Could you check a few things on this drawing? It's one solid part, dimensions in mm from its lowest x, y, z. Round coordinates to 2 decimals unless told otherwise and drop trailing zeros. Write each loop counter-clockwise with the first axis right and the second up, starting at its lowest first coordinate (ties: lowest second). Pieces come first, ordered by that corner, then holes. Notation, with made-up numbers: (-13, 55.25) - (8, 55.25) arc R33 cw to (8, 87.25) - close; hole circle Ø7 at (80, 81). An arc over 180 degrees is marked (long way). One line per question, with ' | ' between items. Start each with the question number.
(1) If I drill on L1, parallel to Y at x = 9, z = 1.55; L2, parallel to X at y = 63.5, z = 3.95, over which ranges is the centre line in solid material (lowest first)?
(2) Imagine slicing it at A-A (y = 9). Write out the boundary of the cut face in (x, z).
(3) Will this pin go through, and if not, where does the flat tip stop? pin 1 (5 mm diameter, centred on x = 9, y = 9, fed in from -Z).
(4) Imagine slicing it at C-C (z = 4.05). Write out the boundary of the cut face in (x, y).
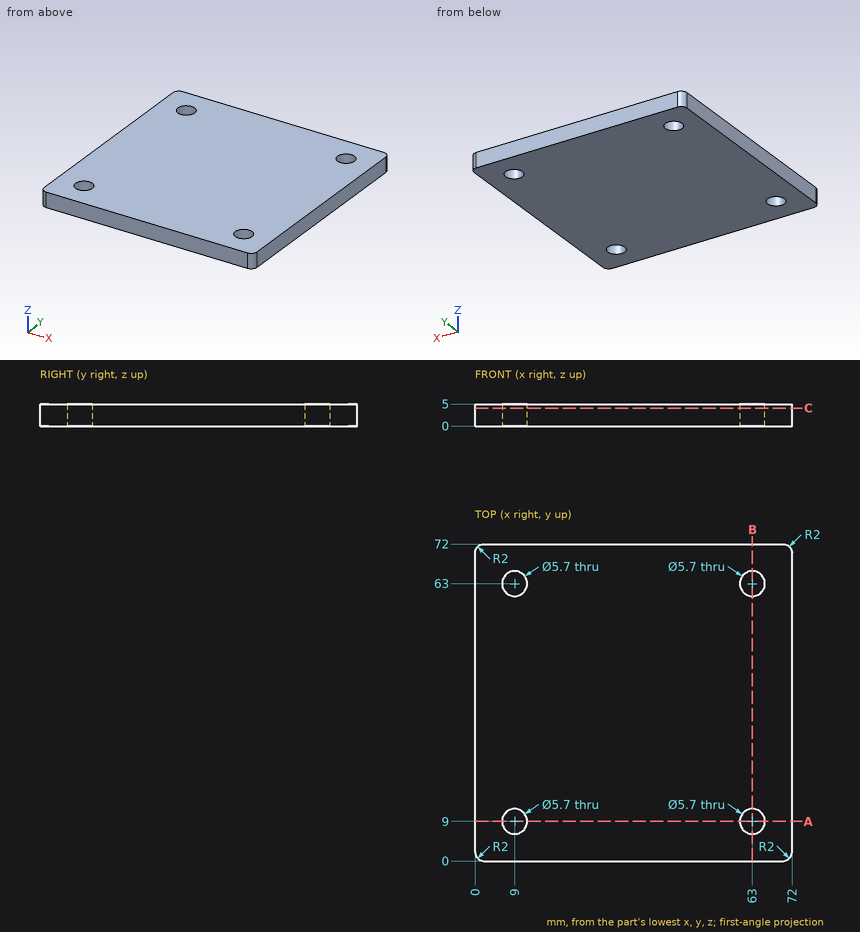
Check sheet entries:
1) L1: 0 to 6.15, 11.85 to 60.15, 65.85 to 72 | L2: 0 to 6.19, 11.81 to 60.19, 65.81 to 72
2) outline: (0, 0) - (6.15, 0) - (6.15, 5) - (0, 5) - close; (11.85, 0) - (60.15, 0) - (60.15, 5) - (11.85, 5) - close; (65.85, 0) - (72, 0) - (72, 5) - (65.85, 5) - close
3) pin 1: through
4) outline: (0, 2) arc R2 ccw to (2, 0) - (70, 0) arc R2 ccw to (72, 2) - (72, 70) arc R2 ccw to (70, 72) - (2, 72) arc R2 ccw to (0, 70) - close; hole circle Ø5.7 at (9, 9); hole circle Ø5.7 at (9, 63); hole circle Ø5.7 at (63, 9); hole circle Ø5.7 at (63, 63)
